from build123d import *

# Parameters (mm, degrees)
MODEL_R             = 1.25
MODEL_W             = 20
MODEL_H             = 3
BOSS_EXTRUDE1_DEPTH = 5


with BuildPart() as part:
    # Model → Boss-Extrude1 (new body)
    with BuildSketch(Plane.XY):
        Polygon((112.443761684, 7.565594359), (132.443761684, 27.565594359), (132.443761684, 57.565594359), (142.443761684, 67.565594359), (142.443761684, 107.565594359), (132.443761684, 117.565594359), (132.443761684, 147.565594359), (112.298529785, 167.710826258), (42.447520771, 167.569353446), (22.443761684, 147.565594359), (22.443761684, 117.565594359), (12.443761684, 107.565594359), (12.443761684, 67.565594359), (22.443761684, 57.565594359), (22.443761684, 27.565594359), (42.443761684, 7.565594359), align=None)
        with Locations((104.943761684, 10.065594359)):
            Circle(MODEL_R, mode=Mode.SUBTRACT)
        with Locations((129.943761684, 35.065594359)):
            Circle(MODEL_R, mode=Mode.SUBTRACT)
        with Locations((120.675994731, 19.333361312)):
            Circle(MODEL_R, mode=Mode.SUBTRACT)
        with Locations((49.943761684, 10.065594359)):
            Circle(MODEL_R, mode=Mode.SUBTRACT)
        with Locations((24.943761684, 35.065594359)):
            Circle(MODEL_R, mode=Mode.SUBTRACT)
        with Locations((34.211528637, 19.333361312)):
            Circle(MODEL_R, mode=Mode.SUBTRACT)
        with Locations((104.943761684, 165.065594359)):
            Circle(MODEL_R, mode=Mode.SUBTRACT)
        with Locations((129.943761684, 140.065594359)):
            Circle(MODEL_R, mode=Mode.SUBTRACT)
        with Locations((120.675994731, 155.797827406)):
            Circle(MODEL_R, mode=Mode.SUBTRACT)
        with Locations((49.943761684, 165.065594359)):
            Circle(MODEL_R, mode=Mode.SUBTRACT)
        with Locations((24.943761684, 140.065594359)):
            Circle(MODEL_R, mode=Mode.SUBTRACT)
        with Locations((34.211528637, 155.797827406)):
            Circle(MODEL_R, mode=Mode.SUBTRACT)
        with Locations((19.211528637, 64.333361312)):
            Circle(MODEL_R, mode=Mode.SUBTRACT)
        with Locations((14.943761684, 87.565594359)):
            Circle(MODEL_R, mode=Mode.SUBTRACT)
        with Locations((19.211528637, 110.797827406)):
            Circle(MODEL_R, mode=Mode.SUBTRACT)
        with Locations((135.675994731, 64.333361312)):
            Circle(MODEL_R, mode=Mode.SUBTRACT)
        with Locations((139.943761684, 87.565594359)):
            Circle(MODEL_R, mode=Mode.SUBTRACT)
        with Locations((135.675994731, 110.797827406)):
            Circle(MODEL_R, mode=Mode.SUBTRACT)
        with Locations((77.443761684, 134.246405176)):
            Rectangle(MODEL_W, MODEL_H, mode=Mode.SUBTRACT)
        with Locations((77.443761684, 40.923947526)):
            Rectangle(MODEL_W, MODEL_H, mode=Mode.SUBTRACT)
        Polygon((111.546053861, 56.329621407), (114.144130073, 54.829621407), (124.144130073, 72.150129482), (121.546053861, 73.650129482), align=None, mode=Mode.SUBTRACT)
        Polygon((114.169567826, 120.316253805), (111.571491615, 118.816253805), (121.571491615, 101.49574573), (124.169567826, 102.99574573), align=None, mode=Mode.SUBTRACT)
        Polygon((40.717955541, 54.814934913), (43.316031753, 56.314934913), (33.316031753, 73.635442988), (30.717955541, 72.135442988), align=None, mode=Mode.SUBTRACT)
        Polygon((30.717955541, 102.99574573), (33.316031753, 101.49574573), (43.316031753, 118.816253805), (40.717955541, 120.316253805), align=None, mode=Mode.SUBTRACT)
    extrude(amount=BOSS_EXTRUDE1_DEPTH)


solid = part.part
Verification items for the finished model (mm, model axes). A direction names the side the tool comes from. Round coordinates to 2 decimals unless told otherwise and drop trailing zeros. Loops run counter-clockwise (first coordinate to the right, second up) from the corner with the lowest first, then second, coordinate; pieces in that order, holes last. Notation, with made-up numbers: (74.25, -27) - (130.25, -27) arc R29 cw to (130.25, 2) - close; hole circle Ø11 at (10.5, 45.5). An arc over 180 degrees is marked (long way). Use a Markdown table: item, result. Add a question column.
1. Section check B-B, the plane y = 24. Record the boundary of the cut face in (x, z).
2. Access from +Z, -Z, +X, -X, +Y, -Y to the whole of each face (thin tool, end or side, straight path). Record for faces 4 (the face through (77, 89, 5)), 5 (the face through (132.444, 42, 2)), 6 (the face through (38.246, 110.035, 2.465)), 7 (the face through (22.444, 133, 2)).
3. Thickness scan on probe 1 along X at (y, z) = (134, 1.95); probe 2 along Y at (x, z) = (49, 2.9); probe 3 along X at (y, z) = (67, 4.45). Record the ranges inside material, lowest first. Write a range as [from, to].
4. Section check C-C, the plane z = 2.75. Give the number of separate pieces and of enclosed holes in the cut face, plus the area to 3 significant figures.
5. Gauge pin test, flat ends, axial feed: pin 1 (1 mm diameter, centred on x = 115.5, z = 2.5, fed in from +Y); pin 2 (1.5 mm diameter, centred on y = 43.5, z = 2, fed in from +X); pin 3 (2.5 mm diameter, centred on x = 75.5, z = 2.5, fed in from +Y); pin 4 (2 mm diameter, centred on x = 139.94, y = 87.57, fed in from +Z). Record the tip position at first contact, or that the pin passes through.
6. Section check A-A, the plane x = 78.5. Record the boundary of the cut face in (y, z), plus the area to 3 significant figures.
7. Release check for a two-part mould opening along Y. For faces 1 (the face through (77, 42.424, 2)), 2 (the face through (77, 89, 0)), 3 (the face through (77, 7.566, 2)) record: released by +Y, released by -Y, zero draft, split by the parting line, or undercut.
Checks:
| question | item | result |
|---|---|---|
| 1 | outline | (26.01, 0) - (128.88, 0) - (128.88, 5) - (26.01, 5) - close |
| 2 | face 4 | +Z, +X, -X, +Y, -Y |
| 2 | face 5 | +Z, -Z, +X, -Y |
| 2 | face 6 | +Z, -Z |
| 2 | face 7 | +Z, -Z, -X, +Y |
| 3 | probe 1 | x = [22.44, 67.44], [87.44, 132.44] |
| 3 | probe 2 | y = [7.57, 9.25], [10.89, 164.25], [165.89, 167.58] |
| 3 | probe 3 | x = [13.01, 33.68], [37.15, 117.71], [121.17, 141.88] |
| 4 | separate pieces | 1 |
| 4 | enclosed holes | 24 |
| 4 | area | 17,400 mm^2 |
| 5 | pin 1 | stops at y = 165.01 |
| 5 | pin 2 | stops at x = 132.44 |
| 5 | pin 3 | stops at y = 167.64 |
| 5 | pin 4 | passes through |
| 6 | outline | (7.57, 0) - (39.42, 0) - (39.42, 5) - (7.57, 5) - close; (42.42, 0) - (132.75, 0) - (132.75, 5) - (42.42, 5) - close; (135.75, 0) - (167.64, 0) - (167.64, 5) - (135.75, 5) - close |
| 6 | area | 770 mm^2 |
| 7 | face 1 | undercut |
| 7 | face 2 | zero draft |
| 7 | face 3 | released by -Y |
